The listing builds one solid part. Answer for the finished solid, in the listing's coordinates (mm). Face numbers are marked on the shaded views. A direction names the side the tool comes from. Coordinates: 2 decimals unless noted, no trailing zeros. Order: outer loops, then holes, each group sorted by start corner. A loop starts at its lowest first (then second) coordinate and runs counter-clockwise, first axis right, second up. Notation, with made-up numbers: M 79.25,85 L 85.25,85 A24 ccw 85.25,122 Z; hole C -19.75,-1 d3. An arc over 180 degrees is marked long. One line per item, written item: value. Start each with the question number.
Q1. For the marked faces 5, 6 and 7, determine the directions among +Z, -Z, +X, -X, +Y, -Y from which every point of the face is accessible in a straight line to the end or side of a thin tool.
Q2. Each of these flat-tipped pins is pushed along its axis until it touches: pin 1 Ø15 at (x, z) = (15, -17) entering from -Y; pin 2 Ø1 at (x, y) = (-1.5, 16) entering from -Z; pin 3 Ø3.5 at (x, y) = (12.5, 70) entering from +Z; pin 4 Ø12 at (y, z) = (13.5, -2.5) entering from +X. Where does it stop, or does it pass through?
Q3. The part is cut by section A-A on z = -11. Give the vertices of the cut face in (x, y), then the cut area to 3 significant figures.
Q4. The part is cut by section B-B on x = 30. Give the vertices of the cut face in (y, z).
Q5. The part is cut by section C-C on z = 2.5. Give the vertices of the cut face in (x, y).
Q6. Determine the mould class of the marked faces 1, 2, 3 and 4 for opening direction Y: pulls with the +Y half, pulls with the -Y half, needs draft (parallel to the pull), parting line crosses it, or undercut.
Q7. Straight lines are drawn through the part: line 1 along X through (y, z) = (48.5, -19); line 2 along Z through (x, y) = (30, 57.75); line 3 along Y through (x, z) = (15, -13). For each, find the intervals that lie inside material, in ascending order. Write a range as [from, to].
Q8. The part is cut by section D-D on y = 9. Give the vertices of the cut face in (x, z), then the cut area to 3 significant figures.
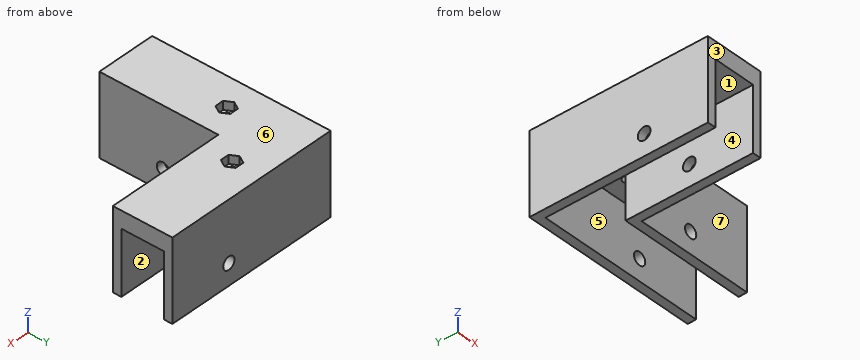
```python
from build123d import *

# Parameters (mm, degrees)
BOSS_EXTRU_1_DEPTH      = 8
ENL_V_MAT_EXTRU_1_DEPTH = 4
ESQUISSE3_R             = 2.25
ENL_V_MAT_EXTRU_2_DEPTH = 5
BOSS_EXTRU_2_DEPTH      = 38
ESQUISSE5_R             = 3
ENL_V_MAT_EXTRU_3_DEPTH = 29
ESQUISSE6_R             = 3
ENL_V_MAT_EXTRU_4_DEPTH = 29


with BuildPart() as part:
    # Esquisse1 → Boss.-Extru.1 (new body)
    with BuildSketch(Plane.XY):
        Polygon((0, 0), (0, 60), (60, 60), (60, 80), (-20, 80), (-20, 0), align=None)
    extrude(amount=BOSS_EXTRU_1_DEPTH)

    # Esquisse2 → Enlèv. mat.-Extru.1 (cut)
    with BuildSketch(Plane.XY.offset(8)):
        Polygon((-14.041451884, 47.5), (-12.020725942, 51), (-7.979274058, 51), (-5.958548116, 47.5), (-7.979274058, 44), (-12.020725942, 44), align=None)
        Polygon((8.458548116, 70), (10.479274058, 73.5), (14.520725942, 73.5), (16.541451884, 70), (14.520725942, 66.5), (10.479274058, 66.5), align=None)
    extrude(amount=-ENL_V_MAT_EXTRU_1_DEPTH, mode=Mode.SUBTRACT)

    # Esquisse3 → Enlèv. mat.-Extru.2 (cut, through all)
    with BuildSketch(Plane.XY.offset(4)):
        with Locations((-10, 47.5)):
            Circle(ESQUISSE3_R)
        with Locations((12.5, 70)):
            Circle(ESQUISSE3_R)
    extrude(amount=-ENL_V_MAT_EXTRU_2_DEPTH, mode=Mode.SUBTRACT)

    # Esquisse4 → Boss.-Extru.2 (add)
    with BuildSketch(Plane.XY.offset(8)):
        Polygon((0, 0), (0, 60), (60, 60), (60, 56), (4, 56), (4, 0), align=None)
        Polygon((60, 80), (60, 84), (-24, 84), (-24, 0), (-20, 0), (-20, 80), align=None)
    extrude(amount=-BOSS_EXTRU_2_DEPTH)

    # Esquisse5 → Enlèv. mat.-Extru.3 (cut, through all)
    with BuildSketch(Plane.XZ.offset(-56)):
        with Locations((30, -20)):
            Circle(ESQUISSE5_R)
    extrude(amount=-ENL_V_MAT_EXTRU_3_DEPTH, mode=Mode.SUBTRACT)

    # Esquisse6 → Enlèv. mat.-Extru.4 (cut, through all)
    with BuildSketch(Plane(origin=(4, 0, 0), x_dir=(0, 0, -1), z_dir=(1, 0, 0))):
        with Locations(Location((20, 30, 0), (0, 0, 90))):  # turned: the seam where the file's is
            Circle(ESQUISSE6_R)
    extrude(amount=-ENL_V_MAT_EXTRU_4_DEPTH, mode=Mode.SUBTRACT)


solid = part.part
```
Output:
1. face 5: -Z, +X
1. face 6: +Z, +X, -X, +Y, -Y
1. face 7: +Z, -Z, +X, -Y
2. pin 1: stops at y = 56
2. pin 2: stops at z = 0
2. pin 3: passes through
2. pin 4: stops at x = 4
3. outline: M -24,0 L -20,0 L -20,80 L 60,80 L 60,84 L -24,84 Z; M 0,0 L 4,0 L 4,56 L 60,56 L 60,60 L 0,60 Z
3. area: 1,120 mm^2
4. outline: M 56,-30 L 60,-30 L 60,-23 L 56,-23 Z; M 56,-17 L 60,-17 L 60,0 L 80,0 L 80,-17 L 84,-17 L 84,8 L 56,8 Z; M 80,-30 L 84,-30 L 84,-23 L 80,-23 Z
5. outline: M -24,0 L 4,0 L 4,56 L 60,56 L 60,84 L -24,84 Z; hole C -10,47.5 d4.5; hole C 12.5,70 d4.5
6. face 1: undercut
6. face 2: undercut
6. face 3: pulls with the -Y half
6. face 4: needs draft
7. line 1: x = [-24, -20], [0, 4]
7. line 2: z = [-30, -23], [-17, 8]
7. line 3: y = [56, 60], [80, 84]
8. outline: M -24,-30 L -20,-30 L -20,0 L 0,0 L 0,-30 L 4,-30 L 4,8 L -24,8 Z
8. area: 464 mm^2
